Geometry check sheet. Reference: the model listing, model coordinates, mm. Give positions to 0.01 mm unless a question says otherwise; leave off trailing zeros. Write each loop counter-clockwise with the first axis right and the second up, starting at its lowest first coordinate (ties: lowest second). Pieces come first, ordered by that corner, then holes.
(1) Mould release check, pull along X, two halves, no side actions. Record for faces 1 (the flat face through (0, 3, -1)), 2 (the flat face through (5, 0, -1)), 3 (the flat face through (10.668, 3, -1)): +X half, -X half, draft (parallel to the pull), parting line (faces both ways), or undercut.
(2) Thickness scan on line 1 along Y through (x, z) = (9, 0.5); line 2 along Z through (x, y) = (3.5, 4.1). Record the ranges inside material, lowest first.
(3) Cross-section at C-C (y = 3.25). Record the boundary of the cut face in (x, z), and give its area (3 significant figures).
(4) Cross-section at A-A (z = 0.5). Count the separate pieces of the cut face and the enclosed holes in it, and give its area (3 significant figures).
(5) Cross-section at B-B (x = 6.75). Record the boundary of the cut face in (y, z), and give its area (3 significant figures).
(6) Cross-section at D-D (x = 8). Record the boundary of the cut face in (y, z).
(7) Depth check by flat-ended pin: P1, Ø0.7, axis at y = 1.5, z = 3, coming from the -X side; P2, Ø0.7, axis at x = 4, z = 5, coming from the +Y side; P3, Ø0.7, axis at y = 1.5, z = 6, coming from the +X side. Enter the tip coordinate at first touch or a pass-through.
Autodesk Inventor part; units mm, degrees
ref_plane "YZ Plane" through (0, 0, 0) normal (1, 0, 0) x (0, 1, 0)
ref_plane "XZ Plane" through (0, 0, 0) normal (0, 1, 0) x (-1, 0, 0)
ref_plane "XY Plane" through (0, 0, 0) normal (0, 0, 1) x (1, 0, 0)
sketch "Sketch1" plane through (0, 0, 0) normal (0, 0, 1) x (1, 0, 0)
  line L0 (0, 5.588) -> (10.668, 5.588)
  line L1 (10.668, 5.588) -> (10.668, 0)
  line L2 (10.668, 0) -> (0, 0)
  line L3 (0, 0) -> (0, 5.588)
  line L4 (9.4615, 4.3815) -> (8.8265, 4.3815)
  line L5 (9.4615, 3.7465) -> (9.4615, 4.3815)
  line L6 (8.8265, 3.7465) -> (9.4615, 3.7465)
  line L7 (8.8265, 4.3815) -> (8.8265, 3.7465)
extrude "Extrusion1" add sketch "Sketch1" against normal blind 2.54
extrude "Extrusion2" add sketch "Sketch1" along normal blind 8.382 contours L5 L6 L7 L4
extrude "Extrusion3" add sketch "Sketch1" against normal blind 5.08 contours L5 L6 L7 L4
pattern_linear "Rectangular Pattern1" count 4 spacing 2.54 along (-1, 0, 0) count 2 spacing 2.54 along (0, -1, 0) of "Extrusion3", "Extrusion2"
properties part number "J23"
Reply:
1. face 1: -X half
1. face 2: draft
1. face 3: +X half
2. line 1: y = 1.21 to 1.84, 3.75 to 4.38
2. line 2: z = -2.54 to 0
3. outline: (0, -2.54) - (10.67, -2.54) - (10.67, 0) - (0, 0) - close
3. area: 27.1 mm2
4. separate pieces: 8
4. enclosed holes: 0
4. area: 3.23 mm2
5. outline: (0, -2.54) - (1.21, -2.54) - (1.21, -5.08) - (1.84, -5.08) - (1.84, -2.54) - (3.75, -2.54) - (3.75, -5.08) - (4.38, -5.08) - (4.38, -2.54) - (5.59, -2.54) - (5.59, 0) - (4.38, 0) - (4.38, 8.38) - (3.75, 8.38) - (3.75, 0) - (1.84, 0) - (1.84, 8.38) - (1.21, 8.38) - (1.21, 0) - (0, 0) - close
5. area: 28.1 mm2
6. outline: (0, -2.54) - (5.59, -2.54) - (5.59, 0) - (0, 0) - close
7. P1: stops at x = 1.21
7. P2: stops at y = 4.38
7. P3: stops at x = 9.46
